```python
from build123d import *

# Parameters (mm, degrees)
BOSS_EXTRUDE1_DEPTH        = 25
F_10_0MM_DOWEL_HOLE1_D     = 10
F_10_0MM_DOWEL_HOLE1_DEPTH = 25
F_10_0MM_DOWEL_HOLE1_TIP   = 3.004303095
SKETCH2_R                  = 6.25
CUT_EXTRUDE2_DEPTH         = 137.504603006
CUT_EXTRUDE3_DEPTH         = 3
CUT_EXTRUDE4_START         = 2.5
CUT_EXTRUDE4_DEPTH         = 20


with BuildPart() as part:
    # Sketch1 → Boss-Extrude1 (new body)
    with BuildSketch(Plane.XY):
        with BuildLine():
            ThreePointArc((3, 75.940766391), (76, 0), (3, -75.940766391))
            Line((3, -75.940766391), (3, -111))
            Line((3, -111), (43, -111))
            Line((43, -111), (43, -82.462112512))
            ThreePointArc((43, -82.462112512), (62.840128265, -68.557408642), (78.41555968, -50))
            Line((78.41555968, -50), (118.41555968, -50))
            Line((118.41555968, -50), (118.41555968, 50))
            Line((118.41555968, 50), (78.41555968, 50))
            ThreePointArc((78.41555968, 50), (62.840128265, 68.557408642), (43, 82.462112512))
            Line((43, 82.462112512), (43, 111))
            Line((43, 111), (3, 111))
            Line((3, 111), (3, 75.940766391))
        make_face()
        with BuildLine():
            ThreePointArc((3, 72.938330115), (73, 0), (3, -72.938330115))
            Line((3, -72.938330115), (3, -75.940766391))
            ThreePointArc((3, -75.940766391), (76, 0), (3, 75.940766391))
            Line((3, 75.940766391), (3, 72.938330115))
        make_face()
    extrude(amount=BOSS_EXTRUDE1_DEPTH)

    # 10.0mm Dowel Hole1
    with Locations(Plane(origin=(118.41555968, 35, 12.5), x_dir=(0, 1, 0), z_dir=(1, 0, 0))):
        with Locations((0, 0), (-69.999928039, 0.100371864)):
            Hole(F_10_0MM_DOWEL_HOLE1_D / 2, depth=F_10_0MM_DOWEL_HOLE1_DEPTH)
            with Locations((0, 0, -(F_10_0MM_DOWEL_HOLE1_DEPTH + F_10_0MM_DOWEL_HOLE1_TIP / 2))):  # 118° drill point
                Cone(0, F_10_0MM_DOWEL_HOLE1_D / 2, F_10_0MM_DOWEL_HOLE1_TIP, mode=Mode.SUBTRACT)

    # Sketch2 → Cut-Extrude2 (cut, through all)
    with BuildSketch(Plane(origin=(43, 0, 0), x_dir=(0, 0, -1), z_dir=(1, 0, 0))):
        with Locations(Location((-12.5, 95, 0), (0, 0, 90))):
            Circle(SKETCH2_R)
        with Locations(Location((-12.5, -95, 0), (0, 0, 90))):
            Circle(SKETCH2_R)
    extrude(amount=-CUT_EXTRUDE2_DEPTH, mode=Mode.SUBTRACT)

    # Sketch2_4 → Cut-Extrude3 (cut)
    with BuildSketch(Plane(origin=(43, 0, 0), x_dir=(0, 0, -1), z_dir=(1, 0, 0))):
        with BuildLine():
            ThreePointArc((-14.5, 86), (-12.5, 84), (-10.5, 86))
            Line((-10.5, 86), (-10.5, 89.078640359))
            ThreePointArc((-10.5, 89.078640359), (-12.5, 88.75), (-14.5, 89.078640359))
            Line((-14.5, 89.078640359), (-14.5, 86))
        make_face()
        with BuildLine():
            ThreePointArc((-10.5, -86), (-12.5, -84), (-14.5, -86))
            Line((-14.5, -86), (-14.5, -89.078640359))
            ThreePointArc((-14.5, -89.078640359), (-12.5, -88.75), (-10.5, -89.078640359))
            Line((-10.5, -89.078640359), (-10.5, -86))
        make_face()
    extrude(amount=-CUT_EXTRUDE3_DEPTH, mode=Mode.SUBTRACT)

    # Sketch1_3 → Cut-Extrude4 (cut)
    with BuildSketch(Plane.XY.offset(CUT_EXTRUDE4_START)):
        with BuildLine():
            ThreePointArc((3, 72.938330115), (73, 0), (3, -72.938330115))
            Line((3, -72.938330115), (3, -75.940766391))
            ThreePointArc((3, -75.940766391), (76, 0), (3, 75.940766391))
            Line((3, 75.940766391), (3, 72.938330115))
        make_face()
    extrude(amount=CUT_EXTRUDE4_DEPTH, mode=Mode.SUBTRACT)


solid = part.part
```
The model under review builds one solid part; all positions refer to its coordinate system, in mm. A direction names the side the tool comes from. Coordinates: 2 decimals unless noted, no trailing zeros. Write each loop counter-clockwise with the first axis right and the second up, starting at its lowest first coordinate (ties: lowest second). Pieces come first, ordered by that corner, then holes.
1) We need section B-B on x = 35.5. State the section outline as (y, z) points.
2) We need section D-D on x = 59.5. State the section outline as (y, z) points.
3) We need section A-A on y = 95. State the section outline as (x, z) points, then the cut area to 3 significant figures.
4) Clearance check with flat-ended pins moving along their axes: pin 1 Ø0.9 at (x, y) = (41.5, -88) entering from -Z; pin 2 Ø1.2 at (y, z) = (-87.5, 12.5) entering from +X; pin 3 Ø2 at (y, z) = (35.5, 10) entering from +X; pin 4 Ø8 at (x, z) = (93, 20) entering from -Y. State where each tip first meets the part, or that it passes through.
5) To check wall thickness, follow probe 1 along Y at (x, z) = (99.5, 12.5); probe 2 along Y at (x, z) = (104, 8.5); probe 3 along Y at (x, z) = (27, 11). State the ranges of each line that lie inside material, in increasing order.
6) We need section C-C on y = 0. State the section outline as (x, z) points, then the cut area to 3 significant figures.
7) The part is to be moulded in two halves that separate along Z. For faces 1 (the face through (72.983, 1.563, 23.732)), 2 (the face through (105.741, 39.995, 12.72)), say which applies: pulls with the +Z half, pulls with the -Z half, needs draft (parallel to the pull), parting line crosses it, or undercut.
8) Machinability: for faces 3 (the face through (23, -111, 12)), 4 (the face through (74, 0, 2.5)), 5 (the face through (99, 50, 12)), 6 (the face through (105.74, -39.62, 10.69)), which of the approach directions +Z, -Z, +X, -X, +Y, -Y give a long, thin tool a straight path to every point of the face, cutting with its end or side? Answer none if there is none.
Answer list:
1. outline: (-111, 0) - (-63.79, 0) - (-63.79, 2.5) - (-67.2, 2.5) - (-67.2, 22.5) - (-63.79, 22.5) - (-63.79, 25) - (-111, 25) - close; (63.79, 0) - (111, 0) - (111, 25) - (63.79, 25) - (63.79, 22.5) - (67.2, 22.5) - (67.2, 2.5) - (63.79, 2.5) - close; hole circle Ø12.5 at (-95, 12.5); hole circle Ø12.5 at (95, 12.5)
2. outline: (-71.48, 0) - (-42.29, 0) - (-42.29, 2.5) - (-47.28, 2.5) - (-47.28, 22.5) - (-42.29, 22.5) - (-42.29, 25) - (-71.48, 25) - close; (42.29, 0) - (71.48, 0) - (71.48, 25) - (42.29, 25) - (42.29, 22.5) - (47.28, 22.5) - (47.28, 2.5) - (42.29, 2.5) - close
3. outline: (3, 0) - (43, 0) - (43, 6.25) - (3, 6.25) - close; (3, 18.75) - (43, 18.75) - (43, 25) - (3, 25) - close
3. area: 500 mm2
4. pin 1: stops at z = 0
4. pin 2: stops at x = 40
4. pin 3: stops at x = 92.54
4. pin 4: stops at y = -50
5. probe 1: y = -50 to -40, -30 to 30, 40 to 50
5. probe 2: y = -50 to -37.86, -32.14 to 32, 38 to 50
5. probe 3: y = -111 to -101.07, -88.93 to -71.04, 71.04 to 88.93, 101.07 to 111
6. outline: (73, 0) - (118.42, 0) - (118.42, 25) - (73, 25) - (73, 22.5) - (76, 22.5) - (76, 2.5) - (73, 2.5) - close
6. area: 1,080 mm2
7. face 1: needs draft
7. face 2: undercut
8. face 3: +Z, -Z, +X, -X, -Y
8. face 4: -X
8. face 5: +Z, -Z, +X, +Y
8. face 6: +X
